Geometry: final body of the model. Coordinates: model frame, mm. A direction names the side the tool comes from. Coordinates: 2 decimals unless noted, no trailing zeros. Write each loop counter-clockwise with the first axis right and the second up, starting at its lowest first coordinate (ties: lowest second). Pieces come first, ordered by that corner, then holes. Notation, with made-up numbers: (62, 47.5) -> (79, 47.5) arc R23 ccw to (79, 72.5) -> close; hole circle Ø3 at (48, 10.5). An arc over 180 degrees is marked (long way). One line per item, written item: value.
```python
from build123d import *

# Parameters (mm, degrees)
ESQUISSE1_R        = 2.500000039
ESQUISSE1_R_2      = 2.5
ESQUISSE1_R_3      = 2.50000052
ESQUISSE1_R_4      = 2.500000067
ESQUISSE1_R_5      = 2
ESQUISSE1_W        = 6
ESQUISSE1_H        = 40
ESQUISSE1_H_2      = 14.000000003
ESQUISSE1_H_3      = 12.5
ESQUISSE1_H_4      = 6
BOSS_EXTRU_1_DEPTH = 6


with BuildPart() as part:
    # Esquisse1 → Boss.-Extru.1 (new body)
    with BuildSketch(Plane.XY):
        Polygon((-395.568859933, 174.308023863), (-401.568859933, 174.308023863), (-401.568859933, 181.409908735), (-465.568859933, 181.409908735), (-465.568859933, 175.409908735), (-485.568859933, 175.409908735), (-485.568859933, 181.409908735), (-501.568859933, 181.409908735), (-527.568859933, 181.409908735), (-527.568859933, 174.308023863), (-521.568859933, 174.308023863), (-521.568859933, 134.309238722), (-527.568859933, 134.309238722), (-527.568859933, 94.307416433), (-521.568859933, 94.307416433), (-521.568859933, 54.308631292), (-527.568859933, 54.308631292), (-527.568859933, 14.306809003), (-521.568859933, 14.306809003), (-521.568859933, -25.691976137), (-527.568859933, -25.691976137), (-527.568859933, -65.693190997), (-501.568859933, -65.693190997), (-501.568859933, -25.693190997), (-495.568859933, -25.693190997), (-495.568859933, -65.693190997), (-485.568859933, -65.693190997), (-485.568859933, -59.693190997), (-465.568859933, -59.693190997), (-465.568859933, -65.693190997), (-401.568859933, -65.693190997), (-401.568859933, -25.691976137), (-395.568859933, -25.691976137), (-395.568859933, 14.306809003), (-401.568859933, 14.306809003), (-401.568859933, 54.308631292), (-395.568859933, 54.308631292), (-395.568859933, 94.307416433), (-401.568859933, 94.307416433), (-401.568859933, 134.309238722), (-395.568859933, 134.309238722), align=None)
        with Locations((-491.068859894, 57.306809003)):
            Circle(ESQUISSE1_R, mode=Mode.SUBTRACT)
        with Locations((-491.068859933, 109.306809003)):
            Circle(ESQUISSE1_R_2, mode=Mode.SUBTRACT)
        with Locations((-429.068859933, 109.306809003)):
            Circle(ESQUISSE1_R_3, mode=Mode.SUBTRACT)
        with Locations((-429.068859933, 57.306809003)):
            Circle(ESQUISSE1_R_4, mode=Mode.SUBTRACT)
        with Locations((-460.068859933, 170.159908735)):
            Circle(ESQUISSE1_R_5, mode=Mode.SUBTRACT)
        with Locations((-432.48625686, 170.159908735)):
            Circle(ESQUISSE1_R_5, mode=Mode.SUBTRACT)
        with Locations((-460.068859933, -54.443190997)):
            Circle(ESQUISSE1_R_5, mode=Mode.SUBTRACT)
        with Locations((-432.48625686, -54.443190997)):
            Circle(ESQUISSE1_R_5, mode=Mode.SUBTRACT)
        with BuildLine():
            Line((-428.48625686, -39.193190997), (-436.48625686, -39.193190997))
            ThreePointArc((-436.48625686, -39.193190997), (-438.48625686, -41.193190997), (-436.48625686, -43.193190997))
            Line((-436.48625686, -43.193190997), (-428.48625686, -43.193190997))
            ThreePointArc((-428.48625686, -43.193190997), (-426.48625686, -41.193190997), (-428.48625686, -39.193190997))
        make_face(mode=Mode.SUBTRACT)
        with Locations((-498.568859933, 34.306809003)):
            Rectangle(ESQUISSE1_W, ESQUISSE1_H, mode=Mode.SUBTRACT)
        with Locations((-498.568859933, 114.306809003)):
            Rectangle(ESQUISSE1_W, ESQUISSE1_H, mode=Mode.SUBTRACT)
        with Locations((-474.318859933, 160.306809004)):
            Rectangle(ESQUISSE1_W, ESQUISSE1_H_2, mode=Mode.SUBTRACT)
        with Locations((-474.318859933, 127.056809003)):
            Rectangle(ESQUISSE1_W, ESQUISSE1_H_3, mode=Mode.SUBTRACT)
        with Locations((-474.318859933, 44.409908732)):
            Rectangle(ESQUISSE1_W, ESQUISSE1_H_4, mode=Mode.SUBTRACT)
    extrude(amount=-BOSS_EXTRU_1_DEPTH)


solid = part.part
```
(1) Section B-B (x = -483). Return the cut outline in (y, z).
Responses:
outline: (-59.69, -6) -> (175.41, -6) -> (175.41, 0) -> (-59.69, 0) -> close
(2) First-contact query: pin 1 (3 mm diameter, centred on y = 38, z = -2.5, fed in from +X); pin 2 (1.8 mm diameter, centred on x = -400, z = -4.5, fed in from -Y). Flat tips, straight axial feed; report the tip coordinate or a pass-through.
Responses:
pin 1: stops at x = -401.57
pin 2: stops at y = -25.69
(3) Line query: line 1 (Y direction, x = -432.5, z = -1.75); line 2 (Y direction, x = -401, z = -4); line 3 (Y direction, x = -476, z = -1.45). Output: solid intervals per line, ascending. Write a range as [from, to].
Responses:
line 1: y = [-65.69, -56.44], [-52.44, -43.19], [-39.19, 168.16], [172.16, 181.41]
line 2: y = [-25.69, 14.31], [54.31, 94.31], [134.31, 174.31]
line 3: y = [-59.69, 41.41], [47.41, 120.81], [133.31, 153.31], [167.31, 175.41]
(4) Pull-direction query (Y, two-part tool) for faces 1 (the flat face through (-399, 14.307, -3)), 2 (the flat face through (-499, 94.307, -3)), 3 (the flat face through (-399, 174.308, -3)), 4 (the flat face through (-434, -65.693, -3)); classes: released by +Y, released by -Y, zero draft, split by the parting line, or undercut.
Responses:
face 1: undercut
face 2: undercut
face 3: released by +Y
face 4: released by -Y
(5) Section D-D (z = -3.1). State how many separate pieces and enclosed holes the cut face has, then the cut area to 3 significant figures.
Responses:
separate pieces: 1
enclosed holes: 14
area: 29,800 mm2
(6) Section A-A (y = 118.5). Return the cut outline in (x, z).
Responses:
outline: (-527.57, -6) -> (-501.57, -6) -> (-501.57, 0) -> (-527.57, 0) -> close; (-495.57, -6) -> (-401.57, -6) -> (-401.57, 0) -> (-495.57, 0) -> close
(7) Section C-C (y = -20.5). Return the cut outline in (x, z), then the cut area to 3 significant figures.
Responses:
outline: (-521.57, -6) -> (-395.57, -6) -> (-395.57, 0) -> (-521.57, 0) -> close
area: 756 mm2
(8) Reachability of faces 5 (the flat face through (-476, -59.693, -3)), 6 (the flat face through (-399, 54.309, -3)), 7 (the flat face through (-465.569, 178, -3)), 8 (the flat face through (-474, 167.307, -3)), 9 (the flat face through (-525, 134.309, -3)) from +Z, -Z, +X, -X, +Y, -Y: full face, straight path, thin tool, end or side. Return the list, or none.
Responses:
face 5: +Z, -Z, -Y
face 6: +Z, -Z, +X
face 7: +Z, -Z, +Y
face 8: +Z, -Z
face 9: +Z, -Z, -X
